Part print with two shaded views. Sizes in mm from the minimum x, y, z corner. Round coordinates to 2 decimals unless told otherwise and drop trailing zeros. Write each loop counter-clockwise with the first axis right and the second up, starting at its lowest first coordinate (ties: lowest second). Pieces come first, ordered by that corner, then holes. Notation, with made-up numbers: M -18.75,-28.5 L 34.25,-28.5 A35 ccw 34.25,4.5 Z; hole C -18,8.25 d4. An arc over 180 degrees is marked long. Use one line per item in the form item = value. Start each with the question number.
Item 1: Cut at C-C, the plane x = 56.2. Give the cut face in (y, z).
Item 2: Cut at D-D, the plane x = 3.3. Give the cut face in (y, z), then the cut area to 3 significant figures.
Item 3: Probe L1, parallel to X at y = 9, z = 1.5; L2, parallel to Y at x = 24.35, z = 1.3; L3, parallel to X at y = 2.75, z = 0.4. List the from-to ranges inside material, lowest first.
Item 4: Cut at B-B, the plane z = 1.7. Give the cut face in (x, y), then the cut area to 3 significant figures.
Item 5: Cut at A-A, the plane y = 10. Give the cut face in (x, z).
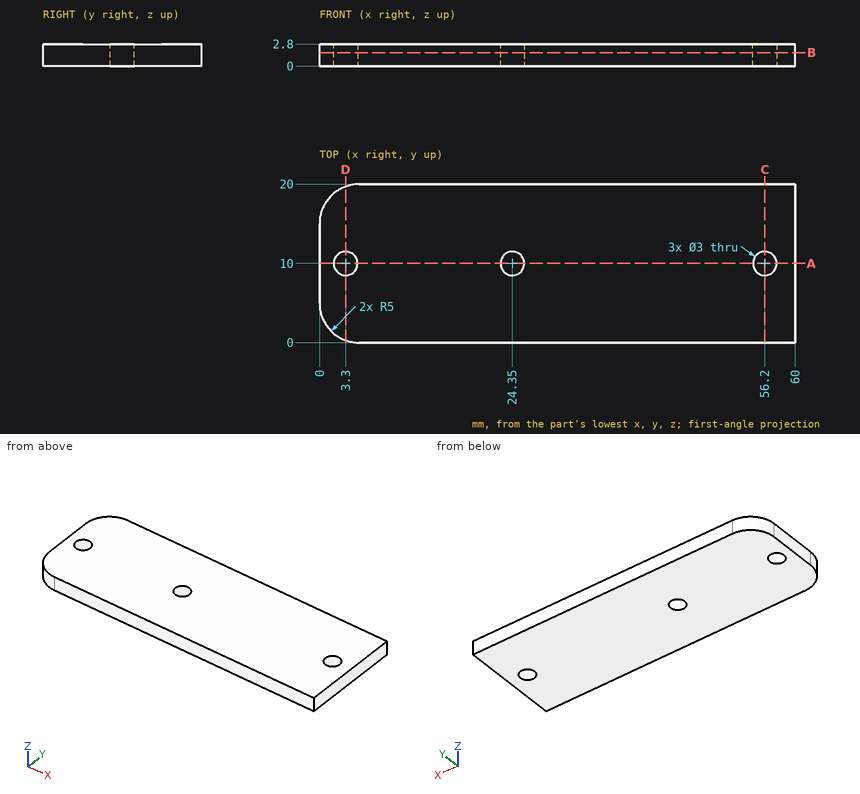
Model answer:
q1.outline = M 0,0 L 8.5,0 L 8.5,2.8 L 0,2.8 Z; M 11.5,0 L 20,0 L 20,2.8 L 11.5,2.8 Z
q2.outline = M 0.3,0 L 8.5,0 L 8.5,2.8 L 0.3,2.8 Z; M 11.5,0 L 19.7,0 L 19.7,2.8 L 11.5,2.8 Z
q2.area = 45.9 mm²
q3.L1 = 0 to 2.18, 4.42 to 23.23, 25.47 to 55.08, 57.32 to 60
q3.L2 = 0 to 8.5, 11.5 to 20
q3.L3 = 0.53 to 60
q4.outline = M 0,5 A5 ccw 5,0 L 60,0 L 60,20 L 5,20 A5 ccw 0,15 Z; hole C 3.3,10 d3; hole C 24.35,10 d3; hole C 56.2,10 d3
q4.area = 1,170 mm²
q5.outline = M 0,0 L 1.8,0 L 1.8,2.8 L 0,2.8 Z; M 4.8,0 L 22.85,0 L 22.85,2.8 L 4.8,2.8 Z; M 25.85,0 L 54.7,0 L 54.7,2.8 L 25.85,2.8 Z; M 57.7,0 L 60,0 L 60,2.8 L 57.7,2.8 Z
